from build123d import *

# Parameters (mm, degrees)
SKETCH1_W                                           = 21
SKETCH1_H                                           = 40
BOSS_EXTRUDE1_DEPTH                                 = 21
SKETCH8_W                                           = 12.85
SKETCH8_H                                           = 12.85
CUT_EXTRUDE2_DEPTH                                  = 40
SKETCH7_W                                           = 12
SKETCH7_H                                           = 30
BOSS_EXTRUDE5_DEPTH                                 = 156
SKETCH9_W                                           = 12
SKETCH9_H                                           = 30
BOSS_EXTRUDE6_DEPTH                                 = 116
SKETCH10_W                                          = 6
SKETCH10_H                                          = 30
BOSS_EXTRUDE7_DEPTH                                 = 20
SKETCH11_W                                          = 7
SKETCH11_H                                          = 30
CUT_EXTRUDE3_DEPTH                                  = 20
CUT_EXTRUDE7_DEPTH                                  = 4.25
CSK_FOR_M4_COUNTERSUNK_FLAT_HEAD_SCREW1_D           = 4.5
CSK_FOR_M4_COUNTERSUNK_FLAT_HEAD_SCREW1_DEPTH       = 16
CSK_FOR_M4_COUNTERSUNK_FLAT_HEAD_SCREW1_CSINK_D     = 9.4
CSK_FOR_M4_COUNTERSUNK_FLAT_HEAD_SCREW1_CSINK_ANGLE = 90
CSK_FOR_M4_COUNTERSUNK_FLAT_HEAD_SCREW1_TIP         = 1.351936393
BOSS_EXTRUDE10_DEPTH                                = 8
BOSS_EXTRUDE11_DEPTH                                = 8
SKETCH27_W                                          = 20
SKETCH27_H                                          = 30
BOSS_EXTRUDE12_DEPTH                                = 1
SKETCH18_R                                          = 2.226933834
CUT_EXTRUDE10_DEPTH                                 = 10.4


with BuildPart() as part:
    # Sketch1 → Boss-Extrude1 (new body)
    with BuildSketch(Plane(origin=(0, 0, 0), x_dir=(0, 0, -1), z_dir=(1, 0, 0))):
        with Locations((2.851327434, 3.994469027)):
            Rectangle(SKETCH1_W, SKETCH1_H)
    extrude(amount=BOSS_EXTRUDE1_DEPTH)

    # Sketch8 → Cut-Extrude2 (cut)
    with BuildSketch(Plane(origin=(0, 23.994469027, 0), x_dir=(1, 0, 0), z_dir=(0, 1, 0))):
        with Locations((10.5, 2.851327434)):
            Rectangle(SKETCH8_W, SKETCH8_H)
    extrude(amount=-CUT_EXTRUDE2_DEPTH, mode=Mode.SUBTRACT)

    # Sketch7 → Boss-Extrude5 (add)
    with BuildSketch(Plane(origin=(0, 0, -13.351327434), x_dir=(-1, 0, 0), z_dir=(0, 0, -1))):
        with Locations((-6, -1.005530973)):
            Rectangle(SKETCH7_W, SKETCH7_H)
    extrude(amount=BOSS_EXTRUDE5_DEPTH)

    # Sketch9 → Boss-Extrude6 (add)
    with BuildSketch(Plane(origin=(21, 0, 0), x_dir=(0, 0, -1), z_dir=(1, 0, 0))):
        with Locations((-1.648672566, -1.005530973)):
            Rectangle(SKETCH9_W, SKETCH9_H)
    extrude(amount=BOSS_EXTRUDE6_DEPTH)

    # Sketch10 → Boss-Extrude7 (add)
    with BuildSketch(Plane(origin=(137, 0, 0), x_dir=(0, 0, -1), z_dir=(1, 0, 0))):
        with Locations((-4.648672566, -1.005530973)):
            Rectangle(SKETCH10_W, SKETCH10_H)
    extrude(amount=BOSS_EXTRUDE7_DEPTH)

    # Sketch11 → Cut-Extrude3 (cut)
    with BuildSketch(Plane(origin=(0, 0, -169.351327434), x_dir=(-1, 0, 0), z_dir=(0, 0, -1))):
        with Locations((-3.5, -1.005530973)):
            Rectangle(SKETCH11_W, SKETCH11_H)
    extrude(amount=-CUT_EXTRUDE3_DEPTH, mode=Mode.SUBTRACT)

    # Sketch16 → Cut-Extrude7 (cut)
    with BuildSketch(Plane(origin=(0, 0, 1.648672566), x_dir=(-1, 0, 0), z_dir=(0, 0, -1))):
        Polygon((-149.064027212, 2.569469027), (-151.128054425, -1.005530973), (-149.064027212, -4.580530973), (-144.935972788, -4.580530973), (-142.871945575, -1.005530973), (-144.935972788, 2.569469027), align=None)
    extrude(amount=-CUT_EXTRUDE7_DEPTH, mode=Mode.SUBTRACT)

    # CSK for M4 Countersunk Flat Head Screw1
    with Locations(Plane(origin=(12, 0, 0), x_dir=(0, 0, 1), z_dir=(1, 0, 0))):
        with Locations((-159.351327434, 1.005530973)):
            CounterSinkHole(CSK_FOR_M4_COUNTERSUNK_FLAT_HEAD_SCREW1_D / 2, CSK_FOR_M4_COUNTERSUNK_FLAT_HEAD_SCREW1_CSINK_D / 2, depth=CSK_FOR_M4_COUNTERSUNK_FLAT_HEAD_SCREW1_DEPTH, counter_sink_angle=CSK_FOR_M4_COUNTERSUNK_FLAT_HEAD_SCREW1_CSINK_ANGLE)
            with Locations((0, 0, -(CSK_FOR_M4_COUNTERSUNK_FLAT_HEAD_SCREW1_DEPTH + CSK_FOR_M4_COUNTERSUNK_FLAT_HEAD_SCREW1_TIP / 2))):  # 118° drill point
                Cone(0, CSK_FOR_M4_COUNTERSUNK_FLAT_HEAD_SCREW1_D / 2, CSK_FOR_M4_COUNTERSUNK_FLAT_HEAD_SCREW1_TIP, mode=Mode.SUBTRACT)

    # Sketch24 → Boss-Extrude10 (add)
    with BuildSketch(Plane(origin=(0, -16.005530973, 0), x_dir=(-1, 0, 0), z_dir=(0, -1, 0))):
        Polygon((-21, 13.351327434), (-30, 4.351327434), (-21, 4.351327434), align=None)
    extrude(amount=-BOSS_EXTRUDE10_DEPTH)

    # Sketch25 → Boss-Extrude11 (add)
    with BuildSketch(Plane(origin=(0, -16.005530973, 0), x_dir=(-1, 0, 0), z_dir=(0, -1, 0))):
        Polygon((-21, 13.351327434), (-12, 22.351327434), (-12, 13.351327434), align=None)
    extrude(amount=-BOSS_EXTRUDE11_DEPTH)

    # Sketch27 → Boss-Extrude12 (add)
    with BuildSketch(Plane(origin=(0, 0, 1.648672566), x_dir=(-1, 0, 0), z_dir=(0, 0, -1))):
        with Locations((-147, -1.005530973)):
            Rectangle(SKETCH27_W, SKETCH27_H)
    extrude(amount=BOSS_EXTRUDE12_DEPTH)

    # Sketch18 → Cut-Extrude10 (cut)
    with BuildSketch(Plane(origin=(0, 0, 0.648672566), x_dir=(-1, 0, 0), z_dir=(0, 0, -1))):
        with Locations((-147, -1.005530973)):
            Circle(SKETCH18_R)
    extrude(amount=-CUT_EXTRUDE10_DEPTH, mode=Mode.SUBTRACT)


solid = part.part
Source: CAD feature listing. Evaluate the final solid. Frame: model axes, mm. A direction names the side the tool comes from. Round coordinates to 2 decimals unless told otherwise and drop trailing zeros. Loops run counter-clockwise (first coordinate to the right, second up) from the corner with the lowest first, then second, coordinate; pieces in that order, holes last. Notation, with made-up numbers: (-9.75, 0) - (23.25, 0) arc R21 cw to (23.25, 22) - close; hole circle Ø10 at (4, 52). An arc over 180 degrees is marked (long way). Write item = value, one per line. Start each with the question number.
Item 1: First-contact query: pin 1 Ø9.5 at (x, z) = (4.5, -89) entering from +Y; pin 2 Ø12 at (y, z) = (-7, -84.5) entering from +X; pin 3 Ø6.5 at (y, z) = (-3.5, -1) entering from +X; pin 4 Ø10.5 at (y, z) = (11, -6) entering from +X. Flat tips, straight axial feed; report the tip coordinate or a pass-through.
Item 2: Section query D-D on z = -32. Output: boundary loops of the cut face in (x, y).
Item 3: Reachability of faces 5 (the face through (10, -1, -169.351)), 6 (the face through (149.4, -0.8, 0.649)), 7 (the face through (145, -3, 1.649)), 8 (the face through (16.925, 4, -3)), 9 (the face through (14, -8.006, -16)) from +Z, -Z, +X, -X, +Y, -Y: full face, straight path, thin tool, end or side. Return the list, or none.
Item 4: Mould query, pull axis X, two halves, no side actions, for faces 1 (the face through (0, -1, -70)), 2 (the face through (149.225, -0.908, 6.761)), 3 (the face through (137, -1, -2)), 4 (the face through (77, -1, 7.649)). Classes: released by +X, released by -X, zero draft, split by the parting line, or undercut.
Item 5: Section query B-B on x = 147. Output: boundary loops of the cut face in (y, z), plus the area to 3 significant figures.
Item 6: Section query C-C on y = -11. Output: boundary loops of the cut face in (x, z) (3 decimals).
Item 7: Section query A-A on y = 8.5. Output: boundary loops of the cut face in (x, z) (3 decimals), plus the area to 3 significant figures.
Item 8: Material intervals for line 1 (X direction, y = 7, z = -33.5); line 2 (Z direction, x = 63, y = -8); line 3 (Y direction, x = 147, z = 7.1), sorted ascending.
Results list:
q1.pin_1 = 13.99
q1.pin_2 = 12
q1.pin_3 = 157
q1.pin_4 = 137
q2.outline = (0, -16.01) - (12, -16.01) - (12, 13.99) - (0, 13.99) - close
q3.face_5 = -Z, +X, -X, +Y, -Y
q3.face_6 = -Z, +X, +Y, -Y
q3.face_7 = none
q3.face_8 = +Y, -Y
q3.face_9 = -Z, +X, +Y
q4.face_1 = released by -X
q4.face_2 = undercut
q4.face_3 = released by +X
q4.face_4 = zero draft
q5.outline = (-16.01, 0.65) - (-3.23, 0.65) - (-3.23, 1.65) - (-4.58, 1.65) - (-4.58, 5.9) - (-3.23, 5.9) - (-3.23, 7.65) - (-16.01, 7.65) - close; (1.22, 0.65) - (13.99, 0.65) - (13.99, 7.65) - (1.22, 7.65) - (1.22, 5.9) - (2.57, 5.9) - (2.57, 1.65) - (1.22, 1.65) - close
q5.area = 167 mm²
q6.outline = (0, -149.351) - (7, -149.351) - (7, -169.351) - (12, -169.351) - (12, -22.351) - (30, -4.351) - (137, -4.351) - (137, 0.649) - (157, 0.649) - (157, 7.649) - (0, 7.649) - close; hole (4.075, -9.276) - (16.925, -9.276) - (16.925, 3.574) - (4.075, 3.574) - close
q7.outline = (0, -149.351) - (7, -149.351) - (7, -169.351) - (12, -169.351) - (12, -13.351) - (21, -13.351) - (21, -4.351) - (137, -4.351) - (137, 0.649) - (157, 0.649) - (157, 7.649) - (0, 7.649) - close; hole (4.075, -9.276) - (16.925, -9.276) - (16.925, 3.574) - (4.075, 3.574) - close
q7.area = 3,540 mm²
q8.line_1 = 0 to 12
q8.line_2 = -4.35 to 7.65
q8.line_3 = -16.01 to -3.23, 1.22 to 13.99
